Model file for the job. Use its own axes, mm. Face numbers are marked on the shaded views. A direction names the side the tool comes from. Coordinates: 2 decimals unless noted, no trailing zeros. Write each loop counter-clockwise with the first axis right and the second up, starting at its lowest first coordinate (ties: lowest second). Pieces come first, ordered by that corner, then holes. Notation, with made-up numbers: (-16.75, 71.25) - (18.25, 71.25) arc R9 cw to (18.25, 85.25) - close; hole circle Ø2 at (-9, -4). An arc over 180 degrees is marked (long way). Put each result on its own line as item: value. Start each with the question number.
1. Pull direction Z, two halves, no side cores. Call the marked faces 1, 2 and 3: released by +Z, released by -Z, zero draft, split by the parting line, or undercut.
2. Saw through at B-B, the plane y = 0.5. Write the cut outline in (x, z).
3. Drill centre lines: L1, parallel to X at y = 2.4, z = -1.2; L2, parallel to Z at x = -1.55, y = 2.45; L3, parallel to Z at x = 1.35, y = 2.9. Where is each one in solid material? Low to high. Write a range as from..to.
4. Which spindle directions (+Z, -Z, +X, -X, +Y, -Y) get a long thin tool onto all of the face, cutting with end or side? Do the marked faces 4 and 5. Say none if no direction does.
5. Drop flat-ended pins along their axis: P1, Ø1.5, axis at y = 2, z = 1.5, coming from the +X side; P2, Ø2, axis at x = 1, y = 1, coming from the +Z side; P3, Ø1, axis at y = 3, z = -0.5, coming from the -X side. Give the stop position or say it passes through.
6. Saw through at A-A, the plane y = 1.85. Write the cut outline in (x, z).
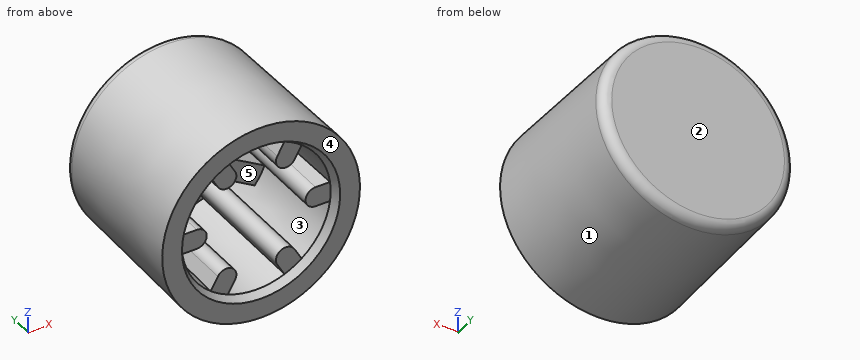
```python
from build123d import *

# Parameters (mm, degrees)
BOSS_EXTRUDE1_DEPTH = 3.25
CIRPATTERN1_COUNT   = 6
BOSS_EXTRUDE2_DEPTH = 0.85
CIRPATTERN2_COUNT   = 3
FILLET1_R           = 0.25


with BuildPart() as part:
    # Sketch1 → Revolve1 (revolve)
    with BuildSketch(Plane.XY, mode=Mode.PRIVATE) as revolve1_sk:
        Polygon((-1.827800985, 3.45), (0, 3.45), (0, 4.03), (-2.429656088, 4.03), (-2.5, 0), (-2, 0), (-1.884529946, 0.2), align=None)
    revolve(revolve1_sk.sketch.rotate(Axis((0, 0, 0), (0, 1, 0)), 270), axis=Axis((0, 0, 0), (0, 1, 0)))

    # Sketch2 → Boss-Extrude1 (add)
    with BuildSketch(Plane.XZ.offset(-3.45)):
        with BuildLine():
            Line((-2, 0.25), (-1.5, 0.25))
            ThreePointArc((-1.5, 0.25), (-1.25, 0), (-1.5, -0.25))
            Line((-1.5, -0.25), (-2, -0.25))
            ThreePointArc((-2, -0.25), (-2.25, 0), (-2, 0.25))
        make_face()
    boss_extrude1 = extrude(amount=BOSS_EXTRUDE1_DEPTH)

    # CirPattern1: Boss-Extrude1 ×6 about axis
    cirpattern1_axis = Axis((0, 0, 0), (0, 1, 0))
    for i in range(1, CIRPATTERN1_COUNT):
        add(boss_extrude1.rotate(cirpattern1_axis, i * 360 / CIRPATTERN1_COUNT))

    # Sketch3 → Boss-Extrude2 (add)
    with BuildSketch(Plane.XZ.offset(-3.45)):
        with BuildLine():
            Line((-0.25, 0.65), (-0.25, 2))
            ThreePointArc((-0.25, 2), (0, 2.25), (0.25, 2))
            Line((0.25, 2), (0.25, 0.65))
            ThreePointArc((0.25, 0.65), (0, 0.4), (-0.25, 0.65))
        make_face()
    boss_extrude2 = extrude(amount=BOSS_EXTRUDE2_DEPTH)

    # CirPattern2: Boss-Extrude2 ×3 about axis
    cirpattern2_axis = Axis((0, 0, 0), (0, 1, 0))
    for i in range(1, CIRPATTERN2_COUNT):
        add(boss_extrude2.rotate(cirpattern2_axis, i * 360 / CIRPATTERN2_COUNT))

    # Fillet1
    fillet1_edges = [part.edges().sort_by_distance(p)[0] for p in [
        (0, 4.03, 2.429656088),
    ]]
    fillet(fillet1_edges, radius=FILLET1_R)


solid = part.part
```
Final values:
1. face 1: split by the parting line
1. face 2: zero draft
1. face 3: undercut
2. outline: circle Ø4.98 at (0, 0); hole (-1.86, -0.25) arc R1.88 ccw to (-1.15, -1.49) - (-0.97, -1.17) arc R0.25 cw to (-0.53, -1.42) - (-0.71, -1.74) arc R1.88 ccw to (0.71, -1.74) - (0.53, -1.42) arc R0.25 cw to (0.97, -1.17) - (1.15, -1.49) arc R1.88 ccw to (1.86, -0.25) - (1.5, -0.25) arc R0.25 cw to (1.5, 0.25) - (1.86, 0.25) arc R1.88 ccw to (1.15, 1.49) - (0.97, 1.17) arc R0.25 cw to (0.53, 1.42) - (0.71, 1.74) arc R1.88 ccw to (-0.71, 1.74) - (-0.53, 1.42) arc R0.25 cw to (-0.97, 1.17) - (-1.15, 1.49) arc R1.88 ccw to (-1.86, 0.25) - (-1.5, 0.25) arc R0.25 cw to (-1.5, -0.25) - close
3. L1: x = -2.15..-1.4, -0.98..-0.52, 0.52..0.98, 1.4..2.15
3. L2: z = -1.91..-1, -0.25..0.25, 1..1.91
3. L3: z = -2.04..-1.25, -1.07..-0.49, -0.2..0.2, 1.25..2.04
4. face 4: +Z, -Z, +X, -X, -Y
4. face 5: -Y
5. P1: stops at x = 2.35
5. P2: stops at z = 2.49
5. P3: stops at x = -2.45
6. outline: circle Ø4.94 at (0, 0); hole (-1.84, -0.25) arc R1.86 ccw to (-1.14, -1.47) - (-0.97, -1.17) arc R0.25 cw to (-0.53, -1.42) - (-0.7, -1.72) arc R1.86 ccw to (0.7, -1.72) - (0.53, -1.42) arc R0.25 cw to (0.97, -1.17) - (1.14, -1.47) arc R1.86 ccw to (1.84, -0.25) - (1.5, -0.25) arc R0.25 cw to (1.5, 0.25) - (1.84, 0.25) arc R1.86 ccw to (1.14, 1.47) - (0.97, 1.17) arc R0.25 cw to (0.53, 1.42) - (0.7, 1.72) arc R1.86 ccw to (-0.7, 1.72) - (-0.53, 1.42) arc R0.25 cw to (-0.97, 1.17) - (-1.14, 1.47) arc R1.86 ccw to (-1.84, 0.25) - (-1.5, 0.25) arc R0.25 cw to (-1.5, -0.25) - close
